Input: part model. Units: mm. Frame: model coordinates. Coordinates: 2 decimals unless noted, no trailing zeros. Order: outer loops, then holes, each group sorted by start corner. A loop starts at its lowest first (then second) coordinate and runs counter-clockwise, first axis right, second up. Notation, with made-up numbers: M -24.75,15 L 20.25,15 A27 cw 20.25,47 Z; hole C 37,-35 d4. An arc over 180 degrees is marked long. One line per item, written item: value.
```python
from build123d import *

# Parameters (mm, degrees)
SKETCH_R     = 9
PAD_DEPTH    = 1
SKETCH001_R  = 3.5
SKETCH002_R  = 3
SKETCH003_R  = 2
POCKET_DEPTH = 7.001


with BuildPart() as pad:
    # Sketch → Pad (new body)
    with BuildSketch(Plane.XY):
        Circle(SKETCH_R)
    extrude(amount=PAD_DEPTH)


with BuildPart() as pocket:
    # Sketch001 → Loft section 0
    with BuildSketch(Plane.XY.offset(1)):
        Circle(SKETCH001_R)
    # Sketch002 → Loft section 1
    with BuildSketch(Plane.XY.offset(7)):
        Circle(SKETCH002_R)
    loft()

    # Fusion: union Pad
    add(pad.part)

    # Sketch003 → Pocket (cut, through all)
    with BuildSketch(Plane.XY.offset(7)):
        Circle(SKETCH003_R)
    extrude(amount=-POCKET_DEPTH, mode=Mode.SUBTRACT)


solid = pocket.part
```
(1) Ray query, line 1 (Z direction, x = 7, y = 2); line 2 (Y direction, x = 0, z = 5.25); line 3 (Y direction, x = 1.75, z = 5). Return the intervals inside material, ascending. Write a range as from..to.
Data:
line 1: z = 0..1
line 2: y = -3.15..-2, 2..3.15
line 3: y = -2.64..-0.97, 0.97..2.64
(2) Cut plane C-C on x = -6. Output: boundary loops of the cut face in (y, z), plus the area to 3 significant figures.
Data:
outline: M -6.71,0 L 6.71,0 L 6.71,1 L -6.71,1 Z
area: 13.4 mm2
(3) Cut plane A-A on x = 0. Output: boundary loops of the cut face in (y, z).
Data:
outline: M -9,0 L -2,0 L -2,7 L -3,7 L -3.5,1 L -9,1 Z; M 2,0 L 9,0 L 9,1 L 3.5,1 L 3,7 L 2,7 Z
(4) First-contact query: pin 1 (1.5 mm diameter, centred on x = -6, z = 3.5, fed in from -Y); pin 2 (5.5 mm diameter, centred on x = 0.5, y = 1.5, fed in from +Z); pin 3 (3 mm diameter, centred on y = 7, z = 1.5, fed in from +X). Flat tips, straight axial feed; report the tip coordinate or a pass-through.
Data:
pin 1: passes through
pin 2: stops at z = 7
pin 3: stops at x = 7.06
(5) Cut plane B-B on z = 3.25. Output: boundary loops of the cut face in (x, y) (1 decimal), plus the area to 3 significant figures.
Data:
outline: C 0,0 d6.6; hole C 0,0 d4
area: 21.9 mm2
(6) Draft query along X for faces 1 (the cylindrical face through (0, -2, 4)), 2 (the conical face through (-0.7, -3.17, 4.04)), 3 (the flat face through (0, -4, 1)). Return one class per face: released by +X, released by -X, zero draft, split by the parting line, or undercut.
Data:
face 1: undercut
face 2: split by the parting line
face 3: zero draft
